CAD build for the part. Positions are in the model's coordinates, mm. Face numbers are marked on the shaded views. A direction names the side the tool comes from. Coordinates: 2 decimals unless noted, no trailing zeros. Write each loop counter-clockwise with the first axis right and the second up, starting at its lowest first coordinate (ties: lowest second). Pieces come first, ordered by that corner, then holes. Notation, with made-up numbers: (58, 52) - (100, 52) arc R22 cw to (100, 60) - close; hole circle Ø10 at (-14.5, 25.5). An arc over 180 degrees is marked (long way). Answer in a Markdown table with one row per item. Add a question column.
Q1. Pin check, flat tips, straight feed: pin 1 (5 mm diameter, centred on x = -5.5, y = 27.5, fed in from +Z); pin 2 (12 mm diameter, centred on y = 15, z = -66, fed in from +X); pin 3 (3 mm diameter, centred on y = 36, z = -60.5, fed in from -X); pin 4 (4 mm diameter, centred on x = -3, y = 31, fed in from -Z). Stop position of each tip, or through.
Q2. 3-axis set-ups, long thin cutter, end or side, ignore diameter. For the marked faces 1 and 2: which of +Z, -Z, +X, -X, +Y, -Y reach the whole face in a straight line?
Q3. Band-saw the part on A-A (y = 35.5). List the corners of the cut face in (x, z).
Q4. Drill centre lines: line 1 along Y through (x, z) = (-1.2, -60); line 2 along Z through (x, y) = (-2, 90); line 3 along X through (y, z) = (17, -61.5). Where is each one in solid material? Low to high. Write a range as from..to.
Q5. Band-saw the part on B-B (y = -6.5). List the corners of the cut face in (x, z).
Autodesk Inventor part; units mm, degrees
ref_plane "YZ Plane" through (0, 0, 0) normal (1, 0, 0) x (0, 1, 0)
ref_plane "XZ Plane" through (0, 0, 0) normal (0, 1, 0) x (-1, 0, 0)
ref_plane "XY Plane" through (0, 0, 0) normal (0, 0, 1) x (1, 0, 0)
sketch "スケッチ2" plane through (0, 0, 0) normal (1, 0, 0) x (0, 1, 0)
  line L0 (0, 0) -> (0, -120)
  line L1 (0, -120) -> (-10, -120)
  line L2 (0, 0) -> (-10, 0)
  line L3 (0, -60) -> (-25, -60)
  arc A0 (-10, 0) -> (-10, -120) centre (102.5, -60) ccw
  line L4 (150, 222.8516) -> (150, -392.0935)
  dimension "d14" = 120
  dimension "d15" = 10
  dimension "d16" = 10
  dimension "d17" = 25
  dimension "d18" = 300
revolve "回転2" add sketch "スケッチ2" angle 5 about axis through (0, 150, 222.8516) along (0, 0, -1)
sketch "スケッチ3" plane through (0, -10, -120) normal (1, 0, 0) x (0, 0, -1)
  line L0 (-70, 110) -> (-50, 110)
  line L1 (-50, 110) -> (-50, 10)
  line L2 (-50, 10) -> (-70, 10)
  line L3 (-70, 10) -> (-70, 110)
  line L4 (0, 0) -> (0, 10)
  line L5 (0, 10) -> (-120, 10)
  dimension "d20" = 100
  dimension "d21" = 20
  dimension "d22" = 50
  dimension "d23" = 0
extrude "押し出し1" add sketch "スケッチ3" against normal blind 5
fillet "フィレット2" radius 2 3 edges at (-2.5003, 0.0208, -50) (-5, 0.0834, -60) (-2.5003, 0.0208, -70)
sketch "スケッチ4" plane through (0, -10, -120) normal (1, 0, 0) x (0, 0, -1)
  line L0 (-50, 12) -> (-50, 110)
  line L1 (-50, 110) -> (-70, 110)
  point P0 (-120, 10)
  point P1 (-60, 100)
  dimension "d27" = 10
  dimension "d28" = 10
hole "穴1" at (0, 90, -60) direction (-1, 0, 0) diameter 6 end through all
fillet "フィレット3" radius 10 2 edges at (-2.5, 100, -50) (-2.5, 100, -70)
properties part number "受動歩行"
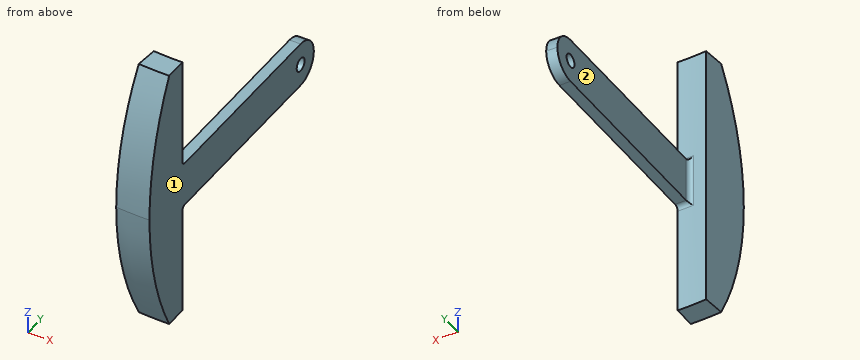
Checked values:
| question | item | result |
|---|---|---|
| 1 | pin 1 | stops at z = -50 |
| 1 | pin 2 | stops at x = 0 |
| 1 | pin 3 | stops at x = -5 |
| 1 | pin 4 | stops at z = -70 |
| 2 | face 1 | +Z, -Z, +X, +Y, -Y |
| 2 | face 2 | +Z, -Z, -X, +Y |
| 3 | outline | (-5, -70) - (0, -70) - (0, -50) - (-5, -50) - close |
| 4 | line 1 | y = -25..87, 93..100 |
| 4 | line 2 | z = -70..-63, -57..-50 |
| 4 | line 3 | x = -5..0 |
| 5 | outline | (-13.69, -120) - (0, -120) - (0, 0) - (-13.69, 0) - close |
